```python
from build123d import *

# Parameters (mm, degrees)
SKETCH1_R                       = 37.5
BOSS_EXTRUDE1_DEPTH             = 37
SKETCH2_R                       = 23.5
CUT_EXTRUDE1_DEPTH              = 22.6
SKETCH3_R                       = 19.5
CUT_EXTRUDE2_DEPTH              = 38
M6X1_0_TAPPED_HOLE1_D           = 5
M6X1_0_TAPPED_HOLE1_DEPTH       = 16
M6X1_0_TAPPED_HOLE1_TIP         = 1.502151548
TAP_DRILL_FOR_M6X1_0_TAP1_D     = 5
TAP_DRILL_FOR_M6X1_0_TAP1_DEPTH = 16
TAP_DRILL_FOR_M6X1_0_TAP1_TIP   = 1.502151548


with BuildPart() as part:
    # Sketch1 → Boss-Extrude1 (new body)
    with BuildSketch(Plane(origin=(0, 0, 0), x_dir=(1, 0, 0), z_dir=(0, 1, 0))):
        Circle(SKETCH1_R)
    extrude(amount=BOSS_EXTRUDE1_DEPTH)

    # Sketch2 → Cut-Extrude1 (cut)
    with BuildSketch(Plane(origin=(0, 37, 0), x_dir=(1, 0, 0), z_dir=(0, 1, 0))):
        Circle(SKETCH2_R)
    extrude(amount=-CUT_EXTRUDE1_DEPTH, mode=Mode.SUBTRACT)

    # Sketch3 → Cut-Extrude2 (cut, through all)
    with BuildSketch(Plane.XZ):
        Circle(SKETCH3_R)
    extrude(amount=-CUT_EXTRUDE2_DEPTH, mode=Mode.SUBTRACT)

    # M6x1.0 Tapped Hole1
    with Locations(Plane(origin=(0, 0, 31), x_dir=(0, 0, -1), z_dir=(0, -1, 0))):
        with Locations((0, 0), (15.5, 26.846787517), (46.5, 26.846787517), (62, 0), (46.5, -26.846787517), (15.5, -26.846787517)):
            Hole(M6X1_0_TAPPED_HOLE1_D / 2, depth=M6X1_0_TAPPED_HOLE1_DEPTH)
            with Locations((0, 0, -(M6X1_0_TAPPED_HOLE1_DEPTH + M6X1_0_TAPPED_HOLE1_TIP / 2))):  # 118° drill point
                Cone(0, M6X1_0_TAPPED_HOLE1_D / 2, M6X1_0_TAPPED_HOLE1_TIP, mode=Mode.SUBTRACT)

    # Tap Drill for M6x1.0 Tap1
    with Locations(Plane(origin=(0, 37, -27.5), x_dir=(0, 0, 1), z_dir=(0, 1, 0))):
        with Locations((0, 0), (13.75, 23.815698604), (41.25, 23.815698604), (55, 0), (41.25, -23.815698604), (13.75, -23.815698604)):
            Hole(TAP_DRILL_FOR_M6X1_0_TAP1_D / 2, depth=TAP_DRILL_FOR_M6X1_0_TAP1_DEPTH)
            with Locations((0, 0, -(TAP_DRILL_FOR_M6X1_0_TAP1_DEPTH + TAP_DRILL_FOR_M6X1_0_TAP1_TIP / 2))):  # 118° drill point
                Cone(0, TAP_DRILL_FOR_M6X1_0_TAP1_D / 2, TAP_DRILL_FOR_M6X1_0_TAP1_TIP, mode=Mode.SUBTRACT)


solid = part.part
```
Part model, mm, in its own coordinate system. A direction names the side the tool comes from. Give positions to 0.01 mm unless a question says otherwise; leave off trailing zeros. Write each loop counter-clockwise with the first axis right and the second up, starting at its lowest first coordinate (ties: lowest second). Pieces come first, ordered by that corner, then holes. Notation, with made-up numbers: (57, 29) -> (90, 29) arc R17 ccw to (90, 33) -> close; hole circle Ø11 at (41.5, 79). An arc over 180 degrees is marked (long way). Put each result on its own line as item: value. Start each with the question number.
Item 1: Cut at C-C (z = 8.5). List the corners of the cut face in (x, y), then the cut area to 3 significant figures.
Item 2: Cut at D-D (y = 3). List the corners of the cut face in (x, z).
Item 3: Cut at A-A (z = 0). List the corners of the cut face in (x, y), then the cut area to 3 significant figures.
Item 4: Wall check: L1, parallel to Z at x = 0, y = 30; L2, parallel to Z at x = 0, y = 6.75; L3, parallel to X at y = 33, z = -15. Give the ranges that are in metal, low to high. Write a range as [from, to].
Item 5: Pull direction Z, two halves, no side cores. Call faces 3 (the face through (26.42, 17.24, -15.41)), 4 (the face through (-1, 37, 24)), 5 (the face through (-24.24, 19.76, -13.84)), 6 (the face through (-4.88, 18.24, -37.18)): pulls with the +Z half, pulls with the -Z half, needs draft (parallel to the pull), parting line crosses it, or undercut.
Item 6: Pin check, flat tips, straight feed: pin 1 Ø5 at (x, y) = (28, 11.5) entering from -Z; pin 2 Ø4.5 at (x, z) = (-23.82, -13.75) entering from +Y; pin 3 Ø1 at (y, z) = (4, -22.5) entering from -X. Stop position of each tip, or through.
Item 7: Which spindle directions (+Z, -Z, +X, -X, +Y, -Y) get a long thin tool onto all of the face, cutting with end or side? Do faces 1 (the face through (0, 29, -25)), 2 (the face through (-26.737, 8.112, 13.002)). Say none if no direction does.
Item 8: Cut at B-B (y = 23). List the corners of the cut face in (x, z), then the cut area to 3 significant figures.
Answer list:
1. outline: (-36.52, 0) -> (-17.55, 0) -> (-17.55, 14.4) -> (-21.91, 14.4) -> (-21.91, 37) -> (-36.52, 37) -> close; (17.55, 0) -> (36.52, 0) -> (36.52, 37) -> (21.91, 37) -> (21.91, 14.4) -> (17.55, 14.4) -> close
1. area: 1,210 mm2
2. outline: circle Ø75 at (0, 0); hole circle Ø5 at (-26.85, -15.5); hole circle Ø5 at (-26.85, 15.5); hole circle Ø39 at (0, 0); hole circle Ø5 at (0, -31); hole circle Ø5 at (0, 31); hole circle Ø5 at (26.85, -15.5); hole circle Ø5 at (26.85, 15.5)
3. outline: (-37.5, 0) -> (-19.5, 0) -> (-19.5, 14.4) -> (-23.5, 14.4) -> (-23.5, 37) -> (-37.5, 37) -> close; (19.5, 0) -> (37.5, 0) -> (37.5, 37) -> (23.5, 37) -> (23.5, 14.4) -> (19.5, 14.4) -> close
3. area: 1,150 mm2
4. L1: z = [-37.5, -30], [-25, -23.5], [23.5, 25], [30, 37.5]
4. L2: z = [-37.5, -33.5], [-28.5, -19.5], [19.5, 28.5], [33.5, 37.5]
4. L3: x = [-34.37, -25.98], [-21.65, -18.09], [18.09, 21.65], [25.98, 34.37]
5. face 3: undercut
5. face 4: needs draft
5. face 5: undercut
5. face 6: parting line crosses it
6. pin 1: stops at z = -27.5
6. pin 2: stops at y = 20.85
6. pin 3: stops at x = -30.37
7. face 1: +Y
7. face 2: -Y
8. outline: circle Ø75 at (0, 0); hole circle Ø5 at (-23.82, -13.75); hole circle Ø5 at (-23.82, 13.75); hole circle Ø47 at (0, 0); hole circle Ø5 at (0, -27.5); hole circle Ø5 at (0, 27.5); hole circle Ø5 at (23.82, -13.75); hole circle Ø5 at (23.82, 13.75)
8. area: 2,570 mm2
